```python
from build123d import *

# Parameters (mm, degrees)
SKETCH1_R           = 2.25
BOSS_EXTRUDE1_DEPTH = 2.54
FILLET2_R           = 12.7
FILLET1_R           = 25.4


with BuildPart() as part:
    # Sketch1 → Boss-Extrude1 (new body)
    with BuildSketch(Plane.XY):
        with BuildLine():
            Line((-15.551371247, -28.902434831), (0, -28.902434831))
            Line((0, -28.902434831), (7.55250204, -28.902434831))
            Line((7.55250204, -28.902434831), (7.55250204, 119.888))
            Line((7.55250204, 119.888), (0, 119.888))
            Line((0, 119.888), (-28.801319167, 119.888))
            Line((-28.801319167, 119.888), (-28.801319167, 116.374908255))
            Line((-28.801319167, 116.374908255), (-26.247498299, 116.374908255))
            Line((-26.247498299, 116.374908255), (-11.247498299, 99.374908255))
            Line((-11.247498299, 99.374908255), (-5.147498299, 99.374908255))
            Line((-5.147498299, 99.374908255), (-5.147498299, 20.374908255))
            Line((-5.147498299, 20.374908255), (-11.247498299, 20.374908255))
            Line((-11.247498299, 20.374908255), (-26.247498299, 3.374908255))
            Line((-26.247498299, 3.374908255), (-39.300222509, 3.374908255))
            Line((-39.300222509, 3.374908255), (-39.300222509, -22.265655957))
            ThreePointArc((-39.300222509, -22.265655957), (-24.907613028, -16.573051533), (-15.551371247, -28.902434831))
        make_face()
        with Locations((-12.247498299, 112.374908255)):
            Circle(SKETCH1_R, mode=Mode.SUBTRACT)
        with Locations((-12.247498299, 7.374908255)):
            Circle(SKETCH1_R, mode=Mode.SUBTRACT)
    extrude(amount=BOSS_EXTRUDE1_DEPTH)

    # Fillet2
    fillet2_edges = [part.edges().sort_by_distance(p)[0] for p in [
        (7.55250204, 119.888, 1.27),
    ]]
    fillet(fillet2_edges, radius=FILLET2_R)

    # Fillet1
    # the kernel refuses this fillet: 25.4 mm, written as the material it takes off along each edge
    with BuildSketch(Plane(origin=(7.55250204, -28.902434831, -63.240009197), x_dir=(0, 1, 0), z_dir=(0, 0, 1))) as fillet1_piece_1:
        with BuildLine():
            CenterArc((25.296003679, 25.4), FILLET1_R, 185.186543812, 84.813456188)
            Line((0, 23.103873287), (-0.505920074, 23.057950753))
            ThreePointArc((-0.505920074, 23.057950753), (-0.508, 11.551936644), (-0.508, 0))
            Line((-0.508, 0), (0, -0.508))
            Line((0, -0.508), (25.296003679, -0.508))
            Line((25.296003679, -0.508), (25.296003679, 0))
        make_face()
    extrude(amount=129.020018394, mode=Mode.SUBTRACT)


solid = part.part
```
Work out the finished part from the listing and answer in its coordinate system (mm). A direction names the side the tool comes from. Round coordinates to 2 decimals unless told otherwise and drop trailing zeros. Write each loop counter-clockwise with the first axis right and the second up, starting at its lowest first coordinate (ties: lowest second). Pieces come first, ordered by that corner, then holes. Notation, with made-up numbers: (-1.5, -35) -> (47.5, -35) arc R15 cw to (47.5, -6) -> close; hole circle Ø4 at (6.25, 46). An arc over 180 degrees is marked (long way). Write each question's results on one line, items separated by ' | '.
Q1. Flat-ended cylindrical pins translate along their axes: P1, Ø1.3, axis at x = -28, z = 1.5, coming from the -Y side; P2, Ø1.3, axis at x = -9.5, z = 1, coming from the -Y side; P3, Ø0.8, axis at y = 76, z = 1, coming from the -X side. Find the tip coordinate at first contact, or state that the pin passes through.
Data:
P1: y = -16.14 | P2: y = -27.81 | P3: x = -5.15
Q2. Which of the six approach directions +Z, -Z, +X, -X, +Y, -Y give full straight-line access (tool end or side, diameter ignored) to faces 5 (the flat face through (-18.85, 107.99, 1.25)), 6 (the flat face through (-28.801, 118, 1)), 7 (the cylindrical face through (-12.54, 114.606, 1.252))?
Data:
face 5: +Z, -Z, -X | face 6: +Z, -Z, -X, +Y | face 7: +Z, -Z
Q3. Section C-C, the plane y = 12 is taken. Write down the section's boundary in (x, z).
Data:
outline: (-18.64, 0) -> (7.55, 0) -> (7.55, 2.54) -> (-18.64, 2.54) -> close
Q4. Section D-D, the plane x = -7.5 is taken. Write down the section's boundary in (y, z).
Data:
outline: (-26.8, 0) -> (20.37, 0) -> (20.37, 2.54) -> (-26.8, 2.54) -> close; (99.37, 0) -> (119.89, 0) -> (119.89, 2.54) -> (99.37, 2.54) -> close
Q5. Section B-B, the plane z = 0.65 is taken. Write down the section's boundary in (x, y).
Data:
outline: (-39.3, -22.27) arc R12.8 cw to (-15.55, -28.9) arc R25.4 ccw to (7.55, -3.61) -> (7.55, 107.19) arc R12.7 ccw to (-5.15, 119.89) -> (-28.8, 119.89) -> (-28.8, 116.37) -> (-26.25, 116.37) -> (-11.25, 99.37) -> (-5.15, 99.37) -> (-5.15, 20.37) -> (-11.25, 20.37) -> (-26.25, 3.37) -> (-39.3, 3.37) -> close; hole circle Ø4.5 at (-12.25, 7.37); hole circle Ø4.5 at (-12.25, 112.37)
Q6. Determine the mould class of faces 1 (the flat face through (-1, 30, 0)), 2 (the cylindrical face through (-25.132, -16.512, 1.252)), 3 (the flat face through (-18.642, 11.994, 1.252)), 4 (the flat face through (-17, 119.888, 1)) for opening direction Y: released by +Y, released by -Y, zero draft, split by the parting line, or undercut.
Data:
face 1: zero draft | face 2: released by -Y | face 3: undercut | face 4: released by +Y
Q7. Section A-A, the plane x = -19 is taken. Write down the section's boundary in (y, z), then the cut area to 3 significant figures.
Data:
outline: (-20.16, 0) -> (11.59, 0) -> (11.59, 2.54) -> (-20.16, 2.54) -> close; (108.16, 0) -> (119.89, 0) -> (119.89, 2.54) -> (108.16, 2.54) -> close | area: 110 mm^2
Q8. Straight lines are drawn through the part: line 1 along X through (y, z) = (82, 1.9); line 2 along X through (y, z) = (-20, 1.45); line 3 along Y through (x, z) = (-9, 2.15). For each, find the intervals that lie inside material, in ascending order. Write a range as [from, to].
Data:
line 1: [-5.15, 7.55] | line 2: [-39.3, -37.55], [-19.15, 1.55] | line 3: [-27.42, 20.37], [99.37, 119.89]
